Source: CAD feature listing. Evaluate the final solid. Frame: model axes, mm. Face numbers are marked on the shaded views. A direction names the side the tool comes from. Give positions to 0.01 mm unless a question says otherwise; leave off trailing zeros. Loops run counter-clockwise (first coordinate to the right, second up) from the corner with the lowest first, then second, coordinate; pieces in that order, holes last.
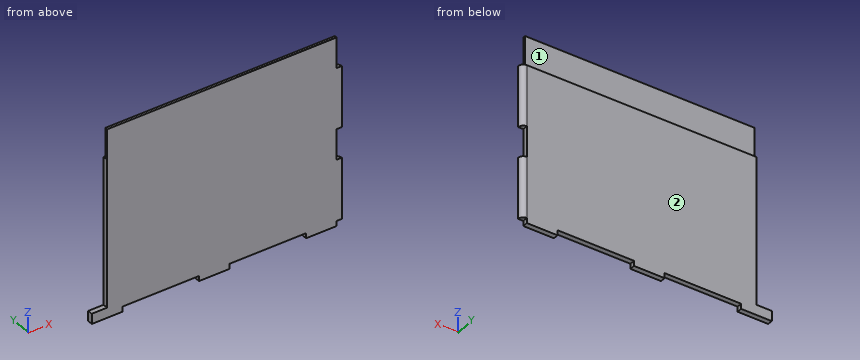
```python
from build123d import *

# Parameters (mm, degrees)
SKETCH_1_W          = 5
SKETCH_1_H          = 60
SKETCH_1_W_2        = 30
SKETCH_1_H_2        = 5
SKETCH_1_W_3        = 15
EXTRUDE_1_DEPTH     = 5
FILLET_1_R          = 5
SKETCH_2_W          = 239.490005879
SKETCH_2_H          = 154.751616696
CUT_EXTRUDE_1_DEPTH = 355.488579047
SKETCH_3_W          = 30
SKETCH_3_H          = 2.5
CUT_EXTRUDE_2_DEPTH = 277.129805813


with BuildPart() as part:
    # 草圖1 → 填料-伸長1 (new body)
    with BuildSketch(Plane(origin=(0, 0, 0), x_dir=(1, 0, 0), z_dir=(0, 1, 0))):
        Polygon((198.746286718, -286.464902661), (198.746286718, -256.464902661), (183.246286718, -256.464902661), (183.246286718, -266.464902661), (124.746286718, -266.464902661), (124.746286718, -262.464902661), (109.246286718, -262.464902661), (109.246286718, -266.464902661), (-21.253713282, -266.464902661), (-21.253713282, 38.535097339), (-36.253713282, 38.535097339), (-36.253713282, 43.535097339), (203.746286718, 43.535097339), (203.746286718, -286.464902661), align=None)
        with Locations((206.246286718, -256.464902661)):
            Rectangle(SKETCH_1_W, SKETCH_1_H)
        with Locations((206.246286718, 13.535097339)):
            Rectangle(SKETCH_1_W, SKETCH_1_H)
        with Locations((188.746286718, 46.035097339)):
            Rectangle(SKETCH_1_W_2, SKETCH_1_H_2)
        with Locations((-21.253713282, 46.035097339)):
            Rectangle(SKETCH_1_W_2, SKETCH_1_H_2)
        with Locations((91.246286718, 46.035097339)):
            Rectangle(SKETCH_1_W_3, SKETCH_1_H_2)
        with Locations((76.246286718, 46.035097339)):
            Rectangle(SKETCH_1_W_3, SKETCH_1_H_2)
        with Locations((206.246286718, -166.464902661)):
            Rectangle(SKETCH_1_W, SKETCH_1_H)
        with Locations((206.246286718, -76.464902661)):
            Rectangle(SKETCH_1_W, SKETCH_1_H)
    extrude(amount=EXTRUDE_1_DEPTH)

    # 圓角1
    fillet_1_edges = [part.edges().sort_by_distance(p)[0] for p in [
        (208.746286718, 5, -13.535097339),
        (208.746286718, 5, 76.464902661),
        (208.746286718, 5, 166.464902661),
        (208.746286718, 5, 256.464902661),
    ]]
    fillet(fillet_1_edges, radius=FILLET_1_R - 0.0001)  # a hair under: the kernel refuses the full size

    # 草圖2 → 除料-伸長1 (cut, through all)
    with BuildSketch(Plane(origin=(0, 5, 0), x_dir=(1, 0, 0), z_dir=(0, 1, 0))):
        with Locations((89.001283779, -213.840711009)):
            Rectangle(SKETCH_2_W, SKETCH_2_H)
    extrude(amount=-CUT_EXTRUDE_1_DEPTH, mode=Mode.SUBTRACT)

    # 草圖3 → 除料-伸長2 (cut, through all)
    with BuildSketch(Plane(origin=(203.746286718, 0, 0), x_dir=(0, 0, -1), z_dir=(1, 0, 0))):
        with Locations((-121.464902661, 3.75)):
            Rectangle(SKETCH_3_W, SKETCH_3_H)
    extrude(amount=-CUT_EXTRUDE_2_DEPTH, mode=Mode.SUBTRACT)


solid = part.part
```
(1) Section B-B, the plane y = 3.85. Return the cut outline in (x, z), then the cut area to 3 significant figures.
A:
outline: (-36.25, -48.54) - (-6.25, -48.54) - (-6.25, -43.54) - (68.75, -43.54) - (68.75, -48.54) - (98.75, -48.54) - (98.75, -43.54) - (173.75, -43.54) - (173.75, -48.54) - (203.75, -48.54) - (203.75, -43.54) - (206.94, -43.54) - (206.94, 16.46) - (203.75, 16.46) - (203.75, 46.46) - (206.94, 46.46) - (206.94, 106.46) - (-21.25, 106.46) - (-21.25, -38.54) - (-36.25, -38.54) - close
area: 34,700 mm2
(2) Reachability of the marked faces 1 and 2 from +Z, -Z, +X, -X, +Y, -Y: full face, straight path, thin tool, end or side. Return the list, or none.
A:
face 1: +Z, +X, -X, +Y
face 2: +Z, -Z, +X, -X, +Y
(3) First-contact query: pin 1 (2.5 mm diameter, centred on y = 3.5, z = -47, fed in from +X); pin 2 (1.5 mm diameter, centred on x = 206.5, y = 1.5, fed in from +Z); pin 3 (2.5 mm diameter, centred on x = 205.5, y = 3.5, fed in from -Z). Flat tips, straight axial feed; report the tip coordinate or a pass-through.
A:
pin 1: stops at x = 203.75
pin 2: stops at z = 106.46
pin 3: stops at z = -43.54
(4) Section A-A, the plane x = 139.5. Return the cut outline in (y, z).
A:
outline: (0, -43.54) - (5, -43.54) - (5, 106.46) - (2.5, 106.46) - (2.5, 136.46) - (0, 136.46) - close
(5) Ray query, line 1 along Z through (x, y) = (164, 2.6); line 2 along Z through (x, y) = (-16.5, 3.25); line 3 along X through (y, z) = (2.3, 44). Return the intervals inside material, ascending.
A:
line 1: z = -43.54 to 106.46
line 2: z = -48.54 to 106.46
line 3: x = -21.25 to 203.75
(6) Section D-D, the plane x = -17. Return the cut outline in (y, z).
A:
outline: (0, -48.54) - (5, -48.54) - (5, 106.46) - (2.5, 106.46) - (2.5, 136.46) - (0, 136.46) - close
